The listing builds one solid part. Answer for the finished solid, in the listing's coordinates (mm). A direction names the side the tool comes from. Give positions to 0.01 mm unless a question says otherwise; leave off trailing zeros. Write each loop counter-clockwise with the first axis right and the second up, starting at its lowest first coordinate (ties: lowest second). Pieces come first, ordered by that corner, then holes. Notation, with made-up numbers: (84, 78) -> (100, 78) arc R20 ccw to (100, 104) -> close; hole circle Ø9 at (-14.5, -38.5). An arc over 180 degrees is marked (long way). One line per question, with ' | ' between items.
from build123d import *

# Parameters (mm, degrees)
SKETCH1_R           = 1
BOSS_EXTRUDE1_DEPTH = 3
SKETCH2_W           = 12.0625
SKETCH2_H           = 66.5
BOSS_EXTRUDE2_DEPTH = 2
FILLET1_R           = 1.5
SKETCH3_W           = 15.875
SKETCH3_H           = 5
SKETCH3_H_2         = 5.08
BOSS_EXTRUDE3_DEPTH = 2
FILLET2_R           = 2.54


with BuildPart() as part:
    # Sketch1 → Boss-Extrude1 (new body)
    with BuildSketch(Plane.XY):
        Polygon((-20, 20), (-20, -20), (-7.9375, -20), (-7.9375, -8.65), (7.9375, -8.65), (7.9375, -20), (20, -20), (20, 20), align=None)
        with Locations((-13.14, -13.14)):
            Circle(SKETCH1_R, mode=Mode.SUBTRACT)
        with Locations((13.14, -13.14)):
            Circle(SKETCH1_R, mode=Mode.SUBTRACT)
        with Locations((-13.14, 13.14)):
            Circle(SKETCH1_R, mode=Mode.SUBTRACT)
        with Locations((13.14, 13.14)):
            Circle(SKETCH1_R, mode=Mode.SUBTRACT)
    extrude(amount=BOSS_EXTRUDE1_DEPTH)

    # Sketch2 → Boss-Extrude2 (add)
    with BuildSketch(Plane.XZ.offset(20)):
        with Locations((-13.96875, -30.25)):
            Rectangle(SKETCH2_W, SKETCH2_H)
        with BuildLine():
            Line((-11.41605, -6.35), (-11.41605, -57.15))
            ThreePointArc((-11.41605, -57.15), (-13.96875, -59.7027), (-16.52145, -57.15))
            Line((-16.52145, -57.15), (-16.52145, -6.35))
            ThreePointArc((-16.52145, -6.35), (-13.96875, -3.7973), (-11.41605, -6.35))
        make_face(mode=Mode.SUBTRACT)
        with Locations((13.96875, -30.25)):
            Rectangle(SKETCH2_W, SKETCH2_H)
        with BuildLine():
            Line((11.41605, -6.35), (11.41605, -57.15))
            ThreePointArc((11.41605, -57.15), (13.96875, -59.7027), (16.52145, -57.15))
            Line((16.52145, -57.15), (16.52145, -6.35))
            ThreePointArc((16.52145, -6.35), (13.96875, -3.7973), (11.41605, -6.35))
        make_face(mode=Mode.SUBTRACT)
    extrude(amount=BOSS_EXTRUDE2_DEPTH)

    # Fillet1
    fillet1_edges = [part.edges().sort_by_distance(p)[0] for p in [
        (13.96875, -20, 0),
        (-13.96875, -20, 0),
    ]]
    fillet(fillet1_edges, radius=FILLET1_R)

    # Sketch3 → Boss-Extrude3 (add)
    with BuildSketch(Plane(origin=(0, -20, 0), x_dir=(1, 0, 0), z_dir=(0, 1, 0))):
        with Locations((0, 61)):
            Rectangle(SKETCH3_W, SKETCH3_H)
        with Locations((0, 32.5)):
            Rectangle(SKETCH3_W, SKETCH3_H_2)
    extrude(amount=-BOSS_EXTRUDE3_DEPTH)

    # Fillet2
    fillet2_edges = [part.edges().sort_by_distance(p)[0] for p in [
        (7.9375, -21, -58.5),
        (-7.9375, -21, -58.5),
        (7.9375, -21, -29.96),
        (7.9375, -21, -35.04),
        (-7.9375, -21, -35.04),
        (-7.9375, -21, -29.96),
    ]]
    fillet(fillet2_edges, radius=FILLET2_R)


solid = part.part
Item 1: Find section C-C (z = -33). Write down the section's boundary in (x, y).
Answers below:
outline: (-20, -22) -> (-16.52, -22) -> (-16.52, -20) -> (-20, -20) -> close; (-11.42, -22) -> (11.42, -22) -> (11.42, -20) -> (-11.42, -20) -> close; (16.52, -22) -> (20, -22) -> (20, -20) -> (16.52, -20) -> close
Item 2: Determine the mould class of faces 4 (the face through (7.938, -20.2, -6.6)), 5 (the face through (0, -22, -31)) for opening direction X: pulls with the +X half, pulls with the -X half, needs draft (parallel to the pull), parting line crosses it, or undercut.
Answers below:
face 4: undercut | face 5: needs draft
Item 3: Find section B-B (x = 4.5). Write down the section's boundary in (y, z).
Answers below:
outline: (-22, -63.5) -> (-20, -63.5) -> (-20, -58.5) -> (-22, -58.5) -> close; (-22, -35.04) -> (-20, -35.04) -> (-20, -29.96) -> (-22, -29.96) -> close; (-8.65, 0) -> (20, 0) -> (20, 3) -> (-8.65, 3) -> close
Item 4: A tool of negligible diameter and unlimited length cuts with its end or side. For faces 1 (the face through (0, -21, -58.5)), 2 (the face through (14.05, -19.57, -0.45)), 3 (the face through (-7.938, -20.2, -6.6)), from which of +Z, -Z, +X, -X, +Y, -Y can it reach the whole face along a straight path? Write none if from no direction.
Answers below:
face 1: +Y, -Y | face 2: -Z, +X, -X, +Y | face 3: +Z, -Y
Item 5: Find section D-D (z = -40.5). Write down the section's boundary in (x, y).
Answers below:
outline: (-20, -22) -> (-16.52, -22) -> (-16.52, -20) -> (-20, -20) -> close; (-11.42, -22) -> (-7.94, -22) -> (-7.94, -20) -> (-11.42, -20) -> close; (7.94, -22) -> (11.42, -22) -> (11.42, -20) -> (7.94, -20) -> close; (16.52, -22) -> (20, -22) -> (20, -20) -> (16.52, -20) -> close
Item 6: Consider line 1 (Y direction, x = -13.14, z = 1.2); line 2 (Y direction, x = 1, z = -32.5); line 3 (Z direction, x = 3, y = 7). Determine where each line is inside the solid, lowest interval first. Write a range as [from, to].
Answers below:
line 1: [-22, -14.14], [-12.14, 12.14], [14.14, 20] | line 2: [-22, -20] | line 3: [0, 3]
Item 7: Flat-ended cylindrical pins translate along their axes: pin 1 (20 mm diameter, centred on x = 3, z = -17.5, fed in from +Y); pin 2 (2 mm diameter, centred on x = -0.5, y = -21, fed in from +Z); pin 3 (3.5 mm diameter, centred on x = -0.5, z = 2, fed in from -Y). Find the tip coordinate at first contact, or state that the pin passes through.
Answers below:
pin 1: y = -20 | pin 2: z = -29.96 | pin 3: y = -8.65
Item 8: Find section A-A (y = -15). Write down the section's boundary in (x, z), then the cut area to 3 significant figures.
Answers below:
outline: (-20, 0) -> (-7.94, 0) -> (-7.94, 3) -> (-20, 3) -> close; (7.94, 0) -> (20, 0) -> (20, 3) -> (7.94, 3) -> close | area: 72.4 mm²
